```python
from build123d import *

# Parameters (mm, degrees)
SKETCH_1_W           = 78
SKETCH_1_H           = 78
EXTRUDE_1_DEPTH      = 5.5
SKETCH_2_W           = 78
SKETCH_2_H           = 78
SKETCH_2_W_2         = 74
SKETCH_2_H_2         = 74
SKETCH_2_W_3         = 5
SKETCH_2_H_3         = 5
EXTRUDE_2_DEPTH      = 10.5
FILLET_1_R           = 1.5
FILLET_2_R           = 3.5
CUT_EXTRUDE_1_DEPTH  = 1
CUT_EXTRUDE_2_DEPTH  = 2.5
SKETCH_5_R           = 1
CUT_EXTRUDE_3_DEPTH  = 58.15767665
CHAMFER_1_SIZE       = 0.5
SKETCH_6_W           = 55
SKETCH_6_H           = 2
SKETCH_6_W_2         = 54
SKETCH_6_H_2         = 58
SKETCH_6_W_3         = 12.5
SKETCH_6_H_3         = 42
CUT_EXTRUDE_4_DEPTH  = 57.553072419
EXTRUDE_3_DEPTH      = 1
EXTRUDE_3_DEPTH_BACK = 2
SKETCH_7_W           = 10
SKETCH_7_H           = 1.5
SKETCH_7_W_2         = 28
SKETCH_8_R           = 4.25
SKETCH_8_R_2         = 2.32594067
CUT_EXTRUDE_5_DEPTH  = 10


with BuildPart() as part:
    # 草图1 → 凸台-拉伸1 (new body)
    with BuildSketch(Plane.XY):
        Rectangle(SKETCH_1_W, SKETCH_1_H)
    extrude(amount=EXTRUDE_1_DEPTH)

    # 草图2 → 凸台-拉伸2 (add)
    # profile 1 of 5: a face of its own
    with BuildSketch(Plane.XY.offset(5.5)):
        Rectangle(SKETCH_2_W, SKETCH_2_H)
        Rectangle(SKETCH_2_W_2, SKETCH_2_H_2, mode=Mode.SUBTRACT)
    # profile 2 of 5: a face of its own
    with BuildSketch(Plane.XY.offset(5.5)):
        with Locations((-34.5, 34.5)):
            Rectangle(SKETCH_2_W_3, SKETCH_2_H_3)
    # profile 3 of 5: a face of its own
    with BuildSketch(Plane.XY.offset(5.5)):
        with Locations((34.5, 34.5)):
            Rectangle(SKETCH_2_W_3, SKETCH_2_H_3)
    # profile 4 of 5: a face of its own
    with BuildSketch(Plane.XY.offset(5.5)):
        with Locations((34.5, -34.5)):
            Rectangle(SKETCH_2_W_3, SKETCH_2_H_3)
    # profile 5 of 5: a face of its own
    with BuildSketch(Plane.XY.offset(5.5)):
        with Locations((-34.5, -34.5)):
            Rectangle(SKETCH_2_W_3, SKETCH_2_H_3)
    extrude(amount=EXTRUDE_2_DEPTH)

    # 圆角1
    fillet_1_edges = [part.edges().sort_by_distance(p)[0] for p in [
        (-37, -32, 10.75),
        (-37, 32, 10.75),
        (-32, 32, 10.75),
        (-32, 37, 10.75),
        (32, 37, 10.75),
        (32, 32, 10.75),
        (37, 32, 10.75),
        (37, -32, 10.75),
        (32, -32, 10.75),
        (32, -37, 10.75),
        (-32, -37, 10.75),
        (-32, -32, 10.75),
    ]]
    fillet(fillet_1_edges, radius=FILLET_1_R)

    # 圆角2
    fillet_2_edges = [part.edges().sort_by_distance(p)[0] for p in [
        (39, -39, 8),
        (-39, -39, 8),
        (-39, 39, 8),
        (39, 39, 8),
    ]]
    fillet(fillet_2_edges, radius=FILLET_2_R)

    # 草图3 → 切除-拉伸1 (cut)
    with BuildSketch(Plane(origin=(0, 0, 0), x_dir=(-1, 0, 0), z_dir=(0, 0, -1))):
        with BuildLine():
            Line((37.5, -35.5), (37.5, 35.5))
            ThreePointArc((37.5, 35.5), (36.914213562, 36.914213562), (35.5, 37.5))
            Line((35.5, 37.5), (-35.5, 37.5))
            ThreePointArc((-35.5, 37.5), (-36.914213562, 36.914213562), (-37.5, 35.5))
            Line((-37.5, 35.5), (-37.5, -35.5))
            ThreePointArc((-37.5, -35.5), (-36.914213562, -36.914213562), (-35.5, -37.5))
            Line((-35.5, -37.5), (35.5, -37.5))
            ThreePointArc((35.5, -37.5), (36.914213562, -36.914213562), (37.5, -35.5))
        make_face()
    extrude(amount=-CUT_EXTRUDE_1_DEPTH, mode=Mode.SUBTRACT)

    # 草图4 → 切除-拉伸2 (cut)
    with BuildSketch(Plane(origin=(0, 0, 1), x_dir=(-1, 0, 0), z_dir=(0, 0, -1))):
        Polygon((27.5, 37.5), (-27.5, 37.5), (-27.5, 36.85), (-32.95, 36.85), (-32.95, -33), (32.95, -33), (32.95, 36.85), (27.5, 36.85), align=None)
    extrude(amount=-CUT_EXTRUDE_2_DEPTH, mode=Mode.SUBTRACT)

    # 草图5 → 切除-拉伸3 (cut, through all)
    with BuildSketch(Plane(origin=(0, 0, 1), x_dir=(-1, 0, 0), z_dir=(0, 0, -1))):
        with Locations((-34.5, 34.5)):
            Circle(SKETCH_5_R)
        with Locations((34.5, 34.5)):
            Circle(SKETCH_5_R)
        with Locations((34.5, -34.5)):
            Circle(SKETCH_5_R)
        with Locations((-34.5, -34.5)):
            Circle(SKETCH_5_R)
    extrude(amount=-CUT_EXTRUDE_3_DEPTH, mode=Mode.SUBTRACT)

    # 倒角1
    chamfer_1_edges = [part.edges().sort_by_distance(p)[0] for p in [
        (-39, 0, 0),
        (39, 0, 0),
        (0, -39, 0),
        (0, 39, 0),
        (-37.974873734, -37.974873734, 0),
        (37.974873734, -37.974873734, 0),
        (37.974873734, 37.974873734, 0),
        (-37.974873734, 37.974873734, 0),
    ]]
    chamfer(chamfer_1_edges, length=CHAMFER_1_SIZE)

    # 草图6 → 切除-拉伸4 (cut, through all)
    with BuildSketch(Plane(origin=(0, 0, 3.5), x_dir=(-1, 0, 0), z_dir=(0, 0, -1))):
        with Locations((0, 36.5)):
            Rectangle(SKETCH_6_W, SKETCH_6_H)
        with Locations((-9, -1)):
            Rectangle(SKETCH_6_W_2, SKETCH_6_H_2)
        with Locations((28.75, 5)):
            Rectangle(SKETCH_6_W_3, SKETCH_6_H_3)
    extrude(amount=-CUT_EXTRUDE_4_DEPTH, mode=Mode.SUBTRACT)

    # 草图7 → 凸台-拉伸3 (add, two sides: drawn at the far end of the back side and taken through both)
    with BuildSketch(Plane.XY.offset(16).offset(-EXTRUDE_3_DEPTH_BACK)):
        with Locations((9, -36.75)):
            Rectangle(SKETCH_7_W, SKETCH_7_H)
        with Locations((-9, -36.75)):
            Rectangle(SKETCH_7_W, SKETCH_7_H)
        with Locations((0, 36.75)):
            Rectangle(SKETCH_7_W_2, SKETCH_7_H)
    extrude(amount=EXTRUDE_3_DEPTH + EXTRUDE_3_DEPTH_BACK)

    # 草图8 → 切除-拉伸5 (cut)
    with BuildSketch(Plane(origin=(39, 0, 0), x_dir=(0, 0, -1), z_dir=(1, 0, 0))):
        with Locations((-15.6, -10.2)):
            Circle(SKETCH_8_R)
        with Locations((-17, 2.7)):
            Circle(SKETCH_8_R_2)
    extrude(amount=-CUT_EXTRUDE_5_DEPTH, mode=Mode.SUBTRACT)


solid = part.part
```
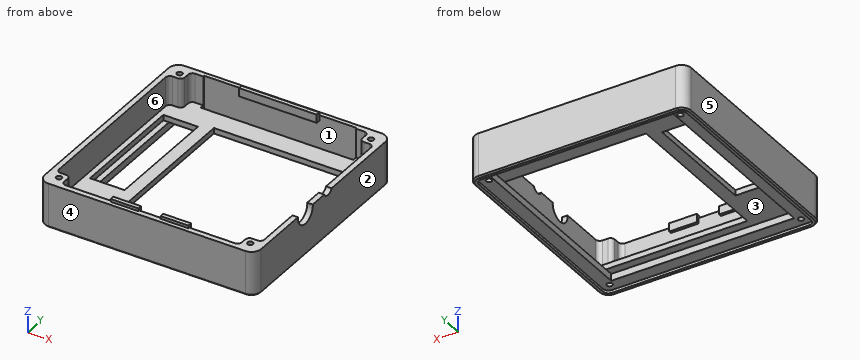
Can you work these out from the model? Positions are in its coordinate system, mm. Face numbers are marked on the shaded views. A direction names the side the tool comes from. Give positions to 0.01 mm unless a question says otherwise; leave off trailing zeros. Order: outer loops, then holes, each group sorted by start corner. A loop starts at its lowest first (then second) coordinate and runs counter-clockwise, first axis right, second up. Notation, with made-up numbers: (10, 37.25) - (64, 37.25) arc R23 ccw to (64, 54.25) - close; hole circle Ø4 at (18, -1). An arc over 180 degrees is marked (long way). Use a Markdown table: item, result. Add a question column.
Q1. If we section it at D-D on x = 2: Write out the boundary of the cut face in (y, z).
Q2. If we section it at A-A on y = 27: Write out the boundary of the cut face in (x, z), plus the area to 3 significant figures.
Q3. On a 3-axis mill with a long thin cutter (end or side, diameter ignored), from which of +Z, -Z, +X, -X, +Y, -Y can I reach the whole of each face in a straight line? I mean the marked faces 5 and 6. Say none if no direction works.
Q4. Please list where these lines run through material, in increasing order: line 1 along Y through (x, z) = (-34.5, 10); line 2 along X through (y, z) = (21, 1.25); line 3 along Y through (x, z) = (-26.5, 6.5).
Q5. I'm going to push flat-ended pins straight in: pin 1 (1.6 mm diameter, centred on y = -36.5, z = 15, fed in from +X); pin 2 (3 mm diameter, centred on x = 34.5, y = 34.5, fed in from -Z); pin 3 (1.6 mm diameter, centred on y = 36.5, z = 5, fed in from -X); pin 4 (1.5 mm diameter, centred on x = 30.5, y = 17.5, fed in from +Z). Where does each tip first touch, or does it pass through?
Q6. If we mould it in two halves opening along X, with no side actions, what happens to the marked faces 1, 2, 3 and 4? For each: released by +X, released by -X, zero draft, split by the parting line, or undercut.
Q7. If we section it at B-B on x = -28.5: Write out the boundary of the cut face in (y, z), plus the area to 3 significant figures.
Q8. If we section it at C-C on y = -10.2: Write out the boundary of the cut face in (x, z), plus the area to 3 significant figures.
Answers follow:
| question | item | result |
|---|---|---|
| 1 | outline | (-39, 0.5) - (-38.5, 0) - (-37.5, 0) - (-37.5, 1) - (-33, 1) - (-33, 3.5) - (-30, 3.5) - (-30, 5.5) - (-37, 5.5) - (-37, 16) - (-39, 16) - close; (28, 3.5) - (35.5, 3.5) - (35.5, 5.5) - (28, 5.5) - close; (36, 14) - (37.5, 14) - (37.5, 0) - (38.5, 0) - (39, 0.5) - (39, 16) - (37.5, 16) - (37.5, 17) - (36, 17) - close |
| 2 | outline | (-39, 0.5) - (-38.5, 0) - (-37.5, 0) - (-37.5, 1) - (-32.95, 1) - (-32.95, 3.5) - (-18, 3.5) - (-18, 5.5) - (-37, 5.5) - (-37, 16) - (-39, 16) - close; (32.95, 1) - (37.5, 1) - (37.5, 0) - (38.5, 0) - (39, 0.5) - (39, 16) - (37, 16) - (37, 5.5) - (36, 5.5) - (36, 3.5) - (32.95, 3.5) - close |
| 2 | area | 123 mm^2 |
| 3 | face 5 | +Z, -Z, -X, +Y, -Y |
| 3 | face 6 | +Z |
| 4 | line 1 | y = -39 to -35.5, -33.5 to -32, 32 to 33.5, 35.5 to 39 |
| 4 | line 2 | x = -39 to -32.95, 32.95 to 39 |
| 4 | line 3 | y = -39 to -37, 37.5 to 39 |
| 5 | pin 1 | stops at x = 38.99 |
| 5 | pin 2 | stops at z = 1 |
| 5 | pin 3 | stops at x = -38.99 |
| 5 | pin 4 | passes through |
| 6 | face 1 | undercut |
| 6 | face 2 | released by +X |
| 6 | face 3 | undercut |
| 6 | face 4 | zero draft |
| 7 | outline | (-39, 0.5) - (-38.5, 0) - (-37.5, 0) - (-37.5, 1) - (-33, 1) - (-33, 3.5) - (-16, 3.5) - (-16, 5.5) - (-37, 5.5) - (-37, 16) - (-39, 16) - close; (26, 3.5) - (36.85, 3.5) - (36.85, 1) - (37.5, 1) - (37.5, 0) - (38.5, 0) - (39, 0.5) - (39, 16) - (37, 16) - (37, 5.5) - (26, 5.5) - close |
| 7 | area | 137 mm^2 |
| 8 | outline | (-39, 0.5) - (-38.5, 0) - (-37.5, 0) - (-37.5, 1) - (-32.95, 1) - (-32.95, 3.5) - (-35, 3.5) - (-35, 5.5) - (-37, 5.5) - (-37, 16) - (-39, 16) - close; (-22.5, 3.5) - (-18, 3.5) - (-18, 5.5) - (-22.5, 5.5) - close; (32.95, 1) - (37.5, 1) - (37.5, 0) - (38.5, 0) - (39, 0.5) - (39, 11.35) - (37, 11.35) - (37, 5.5) - (36, 5.5) - (36, 3.5) - (32.95, 3.5) - close |
| 8 | area | 88.7 mm^2 |
